Design review of the part built by this model. Coordinates are the model's own, in mm. Face numbers are marked on the shaded views. A direction names the side the tool comes from. Give positions to 0.01 mm unless a question says otherwise; leave off trailing zeros. Order: outer loops, then holes, each group sorted by start corner. A loop starts at its lowest first (then second) coordinate and runs counter-clockwise, first axis right, second up. Notation, with made-up numbers: (12.5, 31.5) -> (33.5, 31.5) arc R9 ccw to (33.5, 45.5) -> close; hole circle Ø4 at (54.5, 27). An arc over 180 degrees is marked (long way). One line per item, written item: value.
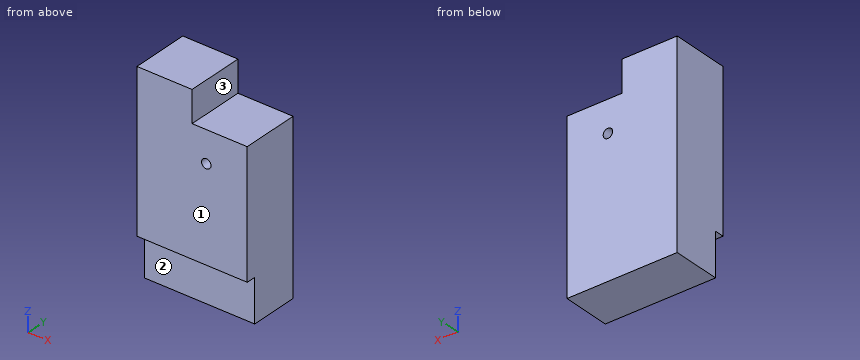
from build123d import *

# Parameters (mm, degrees)
SKETCH_1_W          = 21
SKETCH_1_H          = 38
EXTRUDE_1_DEPTH     = 11
SKETCH_2_W          = 21
SKETCH_2_H          = 8.2
CUT_EXTRUDE_1_DEPTH = 1.8
SKETCH_3_W          = 10.5
SKETCH_3_H          = 11
CUT_EXTRUDE_2_DEPTH = 6
SKETCH_5_R          = 0.9
CUT_EXTRUDE_3_DEPTH = 12


with BuildPart() as part:
    # 草图1 → 凸台-拉伸1 (new body)
    with BuildSketch(Plane(origin=(0, 0, 0), x_dir=(1, 0, 0), z_dir=(0, 1, 0))):
        Rectangle(SKETCH_1_W, SKETCH_1_H)
    extrude(amount=EXTRUDE_1_DEPTH)

    # 草图2 → 切除-拉伸1 (cut)
    with BuildSketch(Plane.XZ):
        with Locations((0, -14.9)):
            Rectangle(SKETCH_2_W, SKETCH_2_H)
    extrude(amount=-CUT_EXTRUDE_1_DEPTH, mode=Mode.SUBTRACT)

    # 草图3 → 切除-拉伸2 (cut)
    with BuildSketch(Plane.XY.offset(19)):
        with Locations((5.25, 5.5)):
            Rectangle(SKETCH_3_W, SKETCH_3_H)
    extrude(amount=-CUT_EXTRUDE_2_DEPTH, mode=Mode.SUBTRACT)

    # 草图5 → 切除-拉伸3 (cut, through all)
    with BuildSketch(Plane(origin=(0, 11, 0), x_dir=(1, 0, 0), z_dir=(0, 1, 0))):
        with Locations((2.7, -7)):
            Circle(SKETCH_5_R)
    extrude(amount=-CUT_EXTRUDE_3_DEPTH, mode=Mode.SUBTRACT)


solid = part.part
Item 1: Add section A-A on z = 7. Give the boundary of the cut face in (x, y), plus the area to 3 significant figures.
Returned:
outline: (-10.5, 0) -> (1.8, 0) -> (1.8, 11) -> (-10.5, 11) -> close; (3.6, 0) -> (10.5, 0) -> (10.5, 11) -> (3.6, 11) -> close
area: 211 mm²
Item 2: Add section B-B on x = 2.7. Give the boundary of the cut face in (y, z).
Returned:
outline: (0, -10.8) -> (1.8, -10.8) -> (1.8, -19) -> (11, -19) -> (11, 6.1) -> (0, 6.1) -> close; (0, 7.9) -> (11, 7.9) -> (11, 13) -> (0, 13) -> close
Item 3: Clearance check with flat-ended pins moving along their axes: P1, Ø0.5, axis at x = 2, y = 1, coming from the -Z side; P2, Ø1, axis at x = 4, y = 3, coming from the +Z side; P3, Ø1.6, axis at x = 2.7, z = 7, coming from the -Y side; P4, Ø4, axis at x = -4, z = -15, coming from the -Y side. State where each tip first meets the part, or that it passes through.
Returned:
P1: z = -10.8
P2: z = 13
P3: through
P4: y = 1.8
Item 4: Add section D-D on y = 0.5. Give the boundary of the cut face in (x, z).
Returned:
outline: (-10.5, -10.8) -> (10.5, -10.8) -> (10.5, 13) -> (0, 13) -> (0, 19) -> (-10.5, 19) -> close; hole circle Ø1.8 at (2.7, 7)
Item 5: To check wall thickness, follow line 1 along X through (y, z) = (3, 7); line 2 along Z through (x, y) = (2.7, 8.5); line 3 along Z through (x, y) = (-9, 1.5). State the ranges of each line that lie inside material, in increasing order. Write a range as from..to.
Returned:
line 1: -10.5..1.8, 3.6..10.5
line 2: -19..6.1, 7.9..13
line 3: -10.8..19
Item 6: Machinability: for the marked faces 1, 2 and 3, which of the approach directions +Z, -Z, +X, -X, +Y, -Y give a long, thin tool a straight path to every point of the face, cutting with its end or side? Answer none if there is none.
Returned:
face 1: +Z, -Z, +X, -X, -Y
face 2: -Z, +X, -X, -Y
face 3: +Z, +X, +Y, -Y
Item 7: Add section C-C on y = 6.25. Give the boundary of the cut face in (x, z), plus the area to 3 significant figures.
Returned:
outline: (-10.5, -19) -> (10.5, -19) -> (10.5, 13) -> (0, 13) -> (0, 19) -> (-10.5, 19) -> close; hole circle Ø1.8 at (2.7, 7)
area: 732 mm²
